```python
from build123d import *

# Parameters (mm, degrees)
SKETCH_1_R                   = 1.5
SKETCH_1_R_2                 = 1.25
EXTRUDE_1_DEPTH              = 7.3
HOLE_WIZARD_M2_51_AT_2_COUNT = 2
HOLE_WIZARD_M2_51_AT_2_PITCH = 10.75


with BuildPart() as part:
    # Эскиз1 → Бобышка-Вытянуть1 (new body)
    with BuildSketch(Plane.XY):
        with BuildLine():
            Line((5, 0), (14.8, 0))
            ThreePointArc((14.8, 0), (18.335533906, 1.464466094), (19.8, 5))
            Line((19.8, 5), (19.8, 16))
            Line((19.8, 16), (0, 16))
            Line((0, 16), (0, 5))
            ThreePointArc((0, 5), (1.464466094, 1.464466094), (5, 0))
        make_face()
        with Locations((9.9, 8)):
            Circle(SKETCH_1_R, mode=Mode.SUBTRACT)
        with Locations((4.525, 11.5)):
            Circle(SKETCH_1_R_2, mode=Mode.SUBTRACT)
        with Locations((4.9, 4)):
            Circle(SKETCH_1_R, mode=Mode.SUBTRACT)
        with Locations((14.9, 4)):
            Circle(SKETCH_1_R, mode=Mode.SUBTRACT)
        with Locations((15.275, 11.5)):
            Circle(SKETCH_1_R_2, mode=Mode.SUBTRACT)
    extrude(amount=-EXTRUDE_1_DEPTH)

    # Эскиз2 → Зенковка для  винта с плоской головкой M2.51 (revolve, cut)
    with BuildSketch(Plane(origin=(4.525, 11.5, 0), x_dir=(0, -1, 0), z_dir=(1, 0, 0))):
        Polygon((0, 0), (0, 7.3), (1.5, 7.3), (1.45, 7.25), (1.45, 0.05), (1.5, 0), align=None)
    hole_wizard_m2_51 = revolve(axis=Axis((4.525, 11.5, 6.35), (0, 0, -1)), mode=Mode.SUBTRACT)

    # Зенковка для  винта с плоской головкой M2.51 at 2: Зенковка для  винта с плоской головкой M2.51 ×2
    with Locations(*[(i * HOLE_WIZARD_M2_51_AT_2_PITCH, 0, 0) for i in range(1, HOLE_WIZARD_M2_51_AT_2_COUNT)]):
        add(hole_wizard_m2_51, mode=Mode.SUBTRACT)


solid = part.part
```
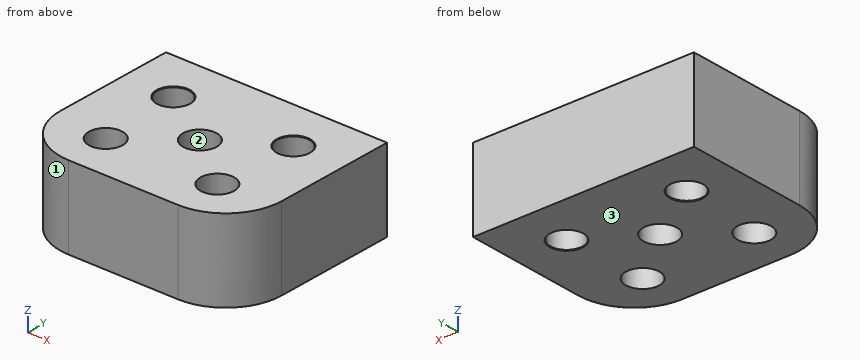
Build history of the part. All positions in model axes, mm. Face numbers are marked on the shaded views. Round coordinates to 2 decimals unless told otherwise and drop trailing zeros. Loops run counter-clockwise (first coordinate to the right, second up) from the corner with the lowest first, then second, coordinate; pieces in that order, holes last.
Item 1: Saw through at A-A (y = 8). List the corners of the cut face in (x, z).
Item 2: Saw through at B-B (x = 9.9). List the corners of the cut face in (y, z), then the cut area to 3 significant figures.
Item 3: Drill centre lines: line 1 along X through (y, z) = (11.5, -4) (3 decimals); line 2 along X through (y, z) = (3.5, -4.75); line 3 along Y through (x, z) = (10.75, -2.5). Where is each one in solid material? Low to high.
Item 4: Saw through at D-D (z = -5.5). List the corners of the cut face in (x, y) (3 decimals), then the cut area to 3 significant figures.
Item 5: Saw through at C-C (y = 4). List the corners of the cut face in (x, z).
Item 6: Two-plate mould, pull along Y, no slides. Class the marked faces 1, 2 and 3: released by +Y, released by -Y, zero draft, split by the parting line, or undercut.
Worked answers:
1. outline: (0, -7.3) - (8.4, -7.3) - (8.4, 0) - (0, 0) - close; (11.4, -7.3) - (19.8, -7.3) - (19.8, 0) - (11.4, 0) - close
2. outline: (0, -7.3) - (6.5, -7.3) - (6.5, 0) - (0, 0) - close; (9.5, -7.3) - (16, -7.3) - (16, 0) - (9.5, 0) - close
2. area: 94.9 mm2
3. line 1: x = 0 to 3.075, 5.975 to 13.825, 16.725 to 19.8
3. line 2: x = 0.23 to 3.49, 6.31 to 13.49, 16.31 to 19.57
3. line 3: y = 0 to 6.76, 9.24 to 16
4. outline: (0, 5) arc R5 ccw to (5, 0) - (14.8, 0) arc R5 ccw to (19.8, 5) - (19.8, 16) - (0, 16) - close; hole circle Ø2.9 at (4.525, 11.5); hole circle Ø3 at (4.9, 4); hole circle Ø3 at (9.9, 8); hole circle Ø3 at (14.9, 4); hole circle Ø2.9 at (15.275, 11.5)
4. area: 272 mm2
5. outline: (0.1, -7.3) - (3.4, -7.3) - (3.4, 0) - (0.1, 0) - close; (6.4, -7.3) - (13.4, -7.3) - (13.4, 0) - (6.4, 0) - close; (16.4, -7.3) - (19.7, -7.3) - (19.7, 0) - (16.4, 0) - close
6. face 1: released by -Y
6. face 2: undercut
6. face 3: zero draft
